The listing builds one solid part. Answer for the finished solid, in the listing's coordinates (mm). A direction names the side the tool comes from. Coordinates: 2 decimals unless noted, no trailing zeros. Order: outer loops, then holes, each group sorted by start corner. A loop starts at its lowest first (then second) coordinate and runs counter-clockwise, first axis right, second up. Notation, with made-up numbers: (-40, 36.5) -> (-22, 36.5) arc R15 cw to (-22, 63.5) -> close; hole circle Ø1 at (-37.5, 9). An arc over 180 degrees is marked (long way). Answer in a Markdown table with one row per item.
```python
from build123d import *

# Parameters (mm, degrees)
F0_R     = 2.5
F1_DEPTH = 54
F2_W     = 12
F2_H     = 40.4068064877
F2_H_2   = 41
F3_DEPTH = 65
F4_R     = 14.3
F5_DEPTH = 100
F7_DEPTH = 100


with BuildPart() as f1:
    # F0 (on Front) → F1 (new body)
    with BuildSketch(Plane.XZ):
        with BuildLine():
            Line((71, 0), (5, 0))
            ThreePointArc((5, 0), (1.4644660941, -1.4644660941), (0, -5))
            Line((0, -5), (0, -58))
            ThreePointArc((0, -58), (1.4644660941, -61.5355339059), (5, -63))
            Line((5, -63), (71, -63))
            ThreePointArc((71, -63), (74.5355339059, -61.5355339059), (76, -58))
            Line((76, -58), (76, -5))
            ThreePointArc((76, -5), (74.5355339059, -1.4644660941), (71, 0))
        make_face()
        with Locations((5, -56)):
            Circle(F0_R, mode=Mode.SUBTRACT)
        with Locations((71, -58)):
            Circle(F0_R, mode=Mode.SUBTRACT)
        with Locations((5, -5)):
            Circle(F0_R, mode=Mode.SUBTRACT)
        with Locations((71, -5)):
            Circle(F0_R, mode=Mode.SUBTRACT)
    extrude(amount=F1_DEPTH)

    # F2 (on Top) → F3 (cut)
    with BuildSketch(Plane.XY):
        with Locations((6, -34.7947494417)):
            Rectangle(F2_W, F2_H)
        with Locations((70.5197853446, -33.6052147746)):
            Rectangle(F2_W, F2_H_2)
    extrude(amount=-F3_DEPTH, mode=Mode.SUBTRACT)

    # F4 (on Right) → F5 (cut)
    with BuildSketch(Plane.YZ):
        with Locations((-32.8, -31.5)):
            Circle(F4_R)
    extrude(amount=F5_DEPTH, mode=Mode.SUBTRACT)

    # F6 (on face) → F7 (cut)
    with BuildSketch(Plane(origin=(12, 0, 0), x_dir=(0, -1, 0), z_dir=(-1, 0, 0))):
        with BuildLine():
            ThreePointArc((42.6762688153, -50.2589795641), (41.5584607083, -50.8062001963), (40.4104675325, -51.2868841392))
            Line((40.4104675325, -51.2868841392), (14.5913461978, -63))
            Line((14.5913461978, -63), (54, -63))
            Line((54, -63), (54, -31.5))
            ThreePointArc((54, -31.5), (50.9496129282, -42.4558911348), (42.6762688153, -50.2589795641))
        make_face()
        with BuildLine():
            ThreePointArc((43.2032697632, -13.0280759466), (51.1028593255, -20.8020870956), (54, -31.5))
            Line((54, -31.5), (54, 0))
            Line((54, 0), (14.5913461978, 0))
            Line((14.5913461978, 0), (39.9029121162, -11.5253000155))
            ThreePointArc((39.9029121162, -11.5253000155), (41.5852822877, -12.205990175), (43.2032697632, -13.0280759466))
        make_face()
    extrude(amount=-F7_DEPTH, mode=Mode.SUBTRACT)


solid = f1.part
```
(1) Find the intervals of material crossed by line 1 along Z through (x, y) = (71, -5); line 2 along Z through (x, y) = (5, -10.25); line 3 along Y through (x, z) = (23, -32), in increasing order. Write a range as from..to.
Check values:
| item | result |
|---|---|
| line 1 | -63..-60.5, -55.5..-7.5, -2.5..0 |
| line 2 | -63..-58.5, -53.5..-7.5, -2.5..0 |
| line 3 | -53.99..-47.09, -18.51..0 |
(2) A cutting plane is placed at D-D, the plane y = -46. Determine the outline of the cut face in (x, z).
Check values:
| item | result |
|---|---|
| outline | (12, -48.09) -> (64.52, -48.09) -> (64.52, -37) -> (12, -37) -> close; (12, -26) -> (64.52, -26) -> (64.52, -14.91) -> (12, -14.91) -> close |
(3) For a pull along Z with two mould halves and no side action, classify faces 1 (the cylindrical face through (2, -7, -1)), 2 (the cylindrical face through (69, -6.5, -6.5)), 3 (the flat face through (64.52, -20, -24)) as released by +Z, released by -Z, zero draft, split by the parting line, or undercut.
Check values:
| item | result |
|---|---|
| face 1 | released by +Z |
| face 2 | undercut |
| face 3 | zero draft |
(4) A cutting plane is placed at C-C, the plane z = -20.5. Determine the outline of the cut face in (x, y), then the cut area to 3 significant figures.
Check values:
| item | result |
|---|---|
| outline | (0, -14.59) -> (12, -14.59) -> (12, -23.66) -> (64.52, -23.66) -> (64.52, -13.11) -> (76, -13.11) -> (76, 0) -> (0, 0) -> close; (12, -50.92) -> (64.52, -50.92) -> (64.52, -41.94) -> (12, -41.94) -> close |
| area | 2,040 mm² |
(5) Flat-ended cylindrical pins translate along their axes: pin 1 (5.5 mm diameter, centred on x = 68.5, z = -30, fed in from -Y); pin 2 (12 mm diameter, centred on x = 47, z = -50, fed in from -Y); pin 3 (5 mm diameter, centred on x = 66, y = -25.5, fed in from +Z). Find the tip coordinate at first contact, or state that the pin passes through.
Check values:
| item | result |
|---|---|
| pin 1 | y = -13.11 |
| pin 2 | y = -49.92 |
| pin 3 | z = -4.05 |
(6) A cutting plane is placed at B-B, the plane y = -11.5. Determine the outline of the cut face in (x, z), then the cut area to 3 significant figures.
Check values:
| item | result |
|---|---|
| outline | (0, -58) arc R5 ccw to (5, -63) -> (71, -63) arc R5 ccw to (76, -58) -> (76, -5) arc R5 ccw to (71, 0) -> (5, 0) arc R5 ccw to (0, -5) -> close; hole circle Ø5 at (5, -56); hole circle Ø5 at (5, -5); hole circle Ø5 at (71, -58); hole circle Ø5 at (71, -5) |
| area | 4,690 mm² |
(7) A cutting plane is placed at A-A, the plane x = 15. Determine the outline of the cut face in (y, z).
Check values:
| item | result |
|---|---|
| outline | (-40.41, -51.29) -> (-14.59, -63) -> (0, -63) -> (0, 0) -> (-14.59, 0) -> (-39.9, -11.53) arc R21.2 ccw to start; hole circle Ø28.6 at (-32.8, -31.5) |
(8) Which of the six approach directions +Z, -Z, +X, -X, +Y, -Y give full straight-line access (tool end or side, diameter ignored) to faces 4 (the flat face through (12, -17, -31)), 5 (the flat face through (70, -13.105, -31)), 6 (the cylindrical face through (69.16, -6.46, -56.31))?
Check values:
| item | result |
|---|---|
| face 4 | +Z, -Z, -X, -Y |
| face 5 | +Z, -Z, +X, -Y |
| face 6 | +Y, -Y |
